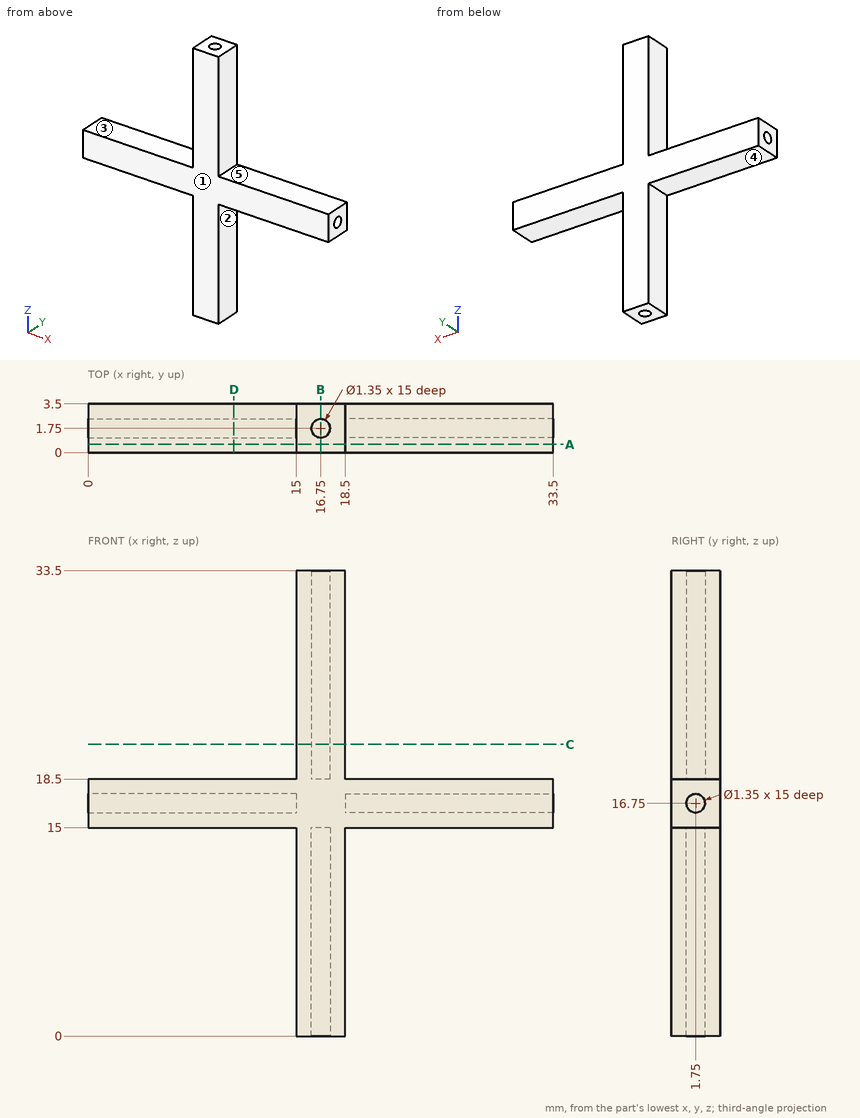
Design review of the part shown in the three views and the two pictorial views. Dimensions are in mm from the part's minimum x, y and z. A direction names the side the tool comes from. Round coordinates to 2 decimals unless told otherwise and drop trailing zeros. Loops run counter-clockwise (first coordinate to the right, second up) from the corner with the lowest first, then second, coordinate; pieces in that order, holes last.
Q1. Insertion check: pin 1 Ø1.8 at (x, y) = (4, 1.5) entering from -Z; pin 2 Ø1 at (y, z) = (2.5, 10) entering from +X; pin 3 Ø1.2 at (x, y) = (16.75, 1.75) entering from +Z. Each pin has a flat end and moves straight along its axis. Give the tip position at first contact, or say it passes through.
Result sheet:
pin 1: stops at z = 15
pin 2: stops at x = 18.5
pin 3: stops at z = 18.5
Q2. Add section D-D on x = 10.5. Write out the cut boundary in (y, z) (3 decimals).
Result sheet:
outline: (0, 15) - (3.5, 15) - (3.5, 18.5) - (0, 18.5) - close; hole circle Ø1.35 at (1.75, 16.75)
Q3. To check wall thickness, follow line 1 along Y through (x, z) = (30.25, 16.75) (3 decimals); line 2 along Z through (x, y) = (5.5, 1.75) (3 decimals); line 3 along X through (y, z) = (1.85, 21.5). State the ranges of each line that lie inside material, in increasing order.
Result sheet:
line 1: y = 0 to 1.075, 2.425 to 3.5
line 2: z = 15 to 16.075, 17.425 to 18.5
line 3: x = 15 to 16.08, 17.42 to 18.5
Q4. Machinability: for the marked faces 1, 2, 3, 4 and 5, which of the approach directions +Z, -Z, +X, -X, +Y, -Y give a long, thin tool a straight path to every point of the face, cutting with its end or side? Answer none if there is none.
Result sheet:
face 1: +Z, -Z, +X, -X, -Y
face 2: -Z, +X, +Y, -Y
face 3: +Z, -X, +Y, -Y
face 4: -Z, -X, +Y, -Y
face 5: +Z, +X, +Y, -Y
Q5. Add section A-A on y = 0.6. Write out the cut boundary in (x, z).
Result sheet:
outline: (0, 15) - (15, 15) - (15, 0) - (18.5, 0) - (18.5, 15) - (33.5, 15) - (33.5, 18.5) - (18.5, 18.5) - (18.5, 33.5) - (15, 33.5) - (15, 18.5) - (0, 18.5) - close
Q6. Add section C-C on z = 21. Write out the cut boundary in (x, y) (3 decimals), plus the area to 3 significant figures.
Result sheet:
outline: (15, 0) - (18.5, 0) - (18.5, 3.5) - (15, 3.5) - close; hole circle Ø1.35 at (16.75, 1.75)
area: 10.8 mm2
Q7. Add section B-B on x = 16.75. Write out the cut boundary in (y, z) (3 decimals).
Result sheet:
outline: (0, 0) - (1.075, 0) - (1.075, 15) - (2.425, 15) - (2.425, 0) - (3.5, 0) - (3.5, 33.5) - (2.425, 33.5) - (2.425, 18.5) - (1.075, 18.5) - (1.075, 33.5) - (0, 33.5) - close
